```python
from build123d import *

# Parameters (mm, degrees)
SKETCH1_W            = 114.3
SKETCH1_H            = 114.3
BASE_EXTRUDE_DEPTH   = 44.45
SKETCH2_R            = 53.975
BOSS_EXTRUDE1_DEPTH  = 304.8
SKETCH3_W            = 114.3
SKETCH3_H            = 114.3
BOSS_EXTRUDE2_DEPTH  = 73.025
SKETCH4_R            = 25.4
BOSS_EXTRUDE3_DEPTH  = 25.4
CUT_EXTRUDE1_START   = -403.225
SKETCH5_R            = 17.4625
CUT_EXTRUDE1_DEPTH   = 403.225
SKETCH6_R            = 4.7625
BOSS_EXTRUDE4_DEPTH  = 361.95
SKETCH7_W            = 193.675
SKETCH7_H            = 114.3
BOSS_EXTRUDE5_DEPTH  = 22.225
CUT_EXTRUDE2_REACH   = 451.274
SKETCH8_R            = 7.9375
LPATTERN2_COUNT      = 2
LPATTERN2_PITCH      = 168.275
LPATTERN2_COUNT_DIR2 = 2
LPATTERN2_PITCH_DIR2 = 88.9


with BuildPart() as part:
    # Sketch1 → Base-Extrude (new body)
    with BuildSketch(Plane(origin=(0, 0, 0), x_dir=(0, 0, -1), z_dir=(1, 0, 0))):
        Rectangle(SKETCH1_W, SKETCH1_H)
    extrude(amount=-BASE_EXTRUDE_DEPTH)

    # Sketch2 → Boss-Extrude1 (add)
    with BuildSketch(Plane.ZY.offset(44.45)):
        with Locations(Location((0, 0, 0), (0, 0, 180))):
            Circle(SKETCH2_R)
    extrude(amount=BOSS_EXTRUDE1_DEPTH)

    # Sketch3 → Boss-Extrude2 (add)
    with BuildSketch(Plane.ZY.offset(349.25)):
        Rectangle(SKETCH3_W, SKETCH3_H)
    extrude(amount=BOSS_EXTRUDE2_DEPTH)

    # Sketch4 → Boss-Extrude3 (add)
    with BuildSketch(Plane.ZY.offset(422.275)):
        with Locations(Location((0, 0, 0), (0, 0, 180))):
            Circle(SKETCH4_R)
    extrude(amount=BOSS_EXTRUDE3_DEPTH)

    # Sketch5 → Cut-Extrude1 (cut)
    with BuildSketch(Plane.ZY.offset(447.675).offset(CUT_EXTRUDE1_START)):
        Circle(SKETCH5_R)
    extrude(amount=CUT_EXTRUDE1_DEPTH, mode=Mode.SUBTRACT)

    # Sketch6 → Boss-Extrude4 (add)
    with BuildSketch(Plane(origin=(-349.25, 0, 0), x_dir=(0, 0, -1), z_dir=(1, 0, 0))):
        with Locations(Location((-44.45, 44.45, 0), (0, 0, 180))):
            Circle(SKETCH6_R)
        with Locations(Location((44.45, 44.45, 0), (0, 0, 180))):
            Circle(SKETCH6_R)
        with Locations(Location((44.45, -44.45, 0), (0, 0, 180))):
            Circle(SKETCH6_R)
        with Locations(Location((-44.45, -44.45, 0), (0, 0, 180))):
            Circle(SKETCH6_R)
    extrude(amount=BOSS_EXTRUDE4_DEPTH)

    # Sketch7 → Boss-Extrude5 (add)
    with BuildSketch(Plane.ZY.offset(422.275)):
        Rectangle(SKETCH7_W, SKETCH7_H)
    extrude(amount=-BOSS_EXTRUDE5_DEPTH)

    # Sketch8 → Cut-Extrude2 (cut, up to next)
    with BuildSketch(Plane.ZY.offset(422.275), mode=Mode.PRIVATE) as cut_extrude2_sk1:
        with Locations((84.1375, -44.45)):
            Circle(SKETCH8_R)
    cut_extrude2_tool1 = extrude(cut_extrude2_sk1.sketch, amount=-CUT_EXTRUDE2_REACH, mode=Mode.PRIVATE) & part.part
    cut_extrude2 = cut_extrude2_tool1.solids().sort_by_distance((-422.275, -44.45, 84.1375))[0]
    add(cut_extrude2, mode=Mode.SUBTRACT)

    # LPattern2: Cut-Extrude2 2 × 2
    with Locations(*[(0, j * LPATTERN2_PITCH_DIR2, -i * LPATTERN2_PITCH) for i in range(LPATTERN2_COUNT) for j in range(LPATTERN2_COUNT_DIR2) if (i, j) != (0, 0)]):
        add(cut_extrude2, mode=Mode.SUBTRACT)


solid = part.part
```
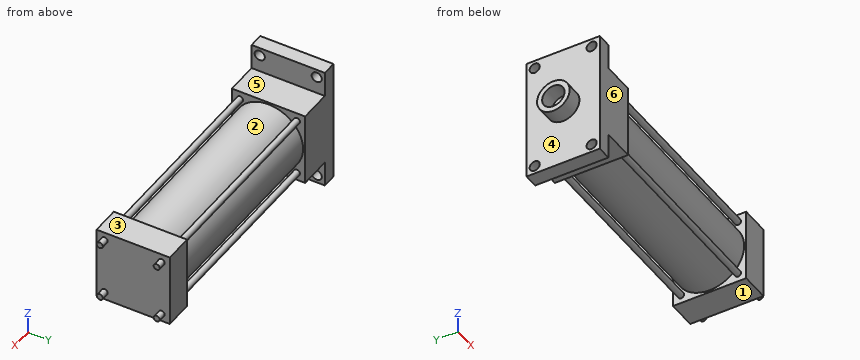
Work out the finished part from the listing and answer in its coordinate system (mm). Face numbers are marked on the shaded views. A direction names the side the tool comes from. Round coordinates to 2 decimals unless told otherwise and drop trailing zeros. One line per question, with ' | ' between items.
Q1. A tool of negligible diameter and unlimited length cuts with its end or side. For the marked faces 5 and 6, from which of +Z, -Z, +X, -X, +Y, -Y can it reach the whole face along a straight path? Write none if from no direction.
Conclusion:
face 5: +Z, +X, +Y, -Y | face 6: +Z, -Z, +X, -X, -Y
Q2. Each of these flat-tipped pins is pushed along its axis until it touches: pin 1 Ø2 at (x, y) = (-338.5, -3.5) entering from -Z; pin 2 Ø1.5 at (y, z) = (-7.5, -35) entering from +X; pin 3 Ø12.5 at (y, z) = (-44.45, -84.14) entering from +X; pin 4 Ø10 at (x, z) = (-96, 48) entering from +Y. Where does it stop, or does it pass through?
Conclusion:
pin 1: stops at z = -53.92 | pin 2: stops at x = 0 | pin 3: passes through | pin 4: stops at y = 49.21
Q3. The mould has two halves that part along Z. Classify the marked faces 1, 2, 3 and 4: +Z half, -Z half, draft (parallel to the pull), parting line (faces both ways), or undercut.
Conclusion:
face 1: -Z half | face 2: undercut | face 3: +Z half | face 4: draft
Q4. Find section B-B, the plane x = -215. State how many separate pieces and enclosed holes the cut face has, then the cut area to 3 significant figures.
Conclusion:
separate pieces: 5 | enclosed holes: 1 | area: 8,480 mm2
Q5. Consider line 1 along Y through (x, z) = (-267, 0) (1 decimal); line 2 along X through (y, z) = (49, -31) (3 decimals); line 3 along Z through (x, y) = (-47, -43). Determine where each line is inside the solid, lowest interval first. Write a range as from..to.
Conclusion:
line 1: y = -54..-17.5, 17.5..54 | line 2: x = -422.275..-349.25, -44.45..0 | line 3: z = -48.99..-39.91, -32.62..32.62, 39.91..48.99
